Check sheet for the modelled part. Datum: model origin and axes. Units: mm. A direction names the side the tool comes from. Give positions to 0.01 mm unless a question says otherwise; leave off trailing zeros. Write each loop counter-clockwise with the first axis right and the second up, starting at its lowest first coordinate (ties: lowest second). Pieces come first, ordered by that corner, then holes. Notation, with made-up numbers: (1.25, 18) - (52.25, 18) arc R11 ccw to (52.25, 39) - close; hole circle Ø8 at (5, 56). An arc over 180 degrees is marked (long way). Return JSON: item names as keys, results as strings. Group by question number.
```python
from build123d import *

# Parameters (mm, degrees)
F0_R        = 19.5387268204
F1_DEPTH    = 101.6
F3_DEPTH    = 38.1
F5_DEPTH    = 25.4
F7_DEPTH    = 25.4
F8_T2_ANGLE = 300.1049055837
F8_T4_ANGLE = 131.5703123603


# Not quite as in the source:
# - a fillet or chamfer that OpenCascade refuses, or shapes differently, is made with other operations: its cross-section is extruded or revolved along the edge and cut away or added


with BuildPart() as f1:
    # F0 (on Right) → F1 (new body, symmetric)
    with BuildSketch(Plane.YZ):
        Circle(F0_R)
    extrude(amount=F1_DEPTH, both=True)

    # F2 (on Top) → F3 (cut)
    with BuildSketch(Plane.XY):
        Polygon((-49.3527501822, 13.7382084504), (-37.9295572639, 12.1708353981), (-49.3527501822, 22.1678428352), align=None)
    extrude(amount=-F3_DEPTH, mode=Mode.SUBTRACT)

    # F4 (on Top) → F5 (cut)
    with BuildSketch(Plane.XY):
        Polygon((-103.1729057431, 0), (-93.9432457089, -16.6200213134), (-87.8715068102, -10.7566714287), align=None)
        Polygon((22.2135502845, -11.3549903035), (22.2135502845, -20.1754160225), (26.9660595804, -20.1754160225), align=None)
        Polygon((-77.9622271657, 12.2874397784), (-86.7114588618, 22.1413038671), (-82.0683091879, 6.1605265364), (-65.0239139795, 12.2874397784), (-72.4504972355, 17.1812968249), align=None)
        Polygon((0, 22.1413038671), (-8.541457355, 12.2874397784), (0, 12.2874397784), align=None)
        Polygon((-27.3653976619, -12.4159986153), (-27.3653976619, -20.1754160225), (-12.2119756415, -16.6692733765), (-18.8832655549, -12.4159986153), align=None)
    extrude(amount=-F5_DEPTH, mode=Mode.SUBTRACT)

    # F6 (on Top) → F7 (cut)
    with BuildSketch(Plane.XY):
        Polygon((-32.052900187, -20.8235712349), (-20.0643315911, -22.1631750464), (-25.0567086041, -9.0359868482), (-35.0853319095, -12.8499542954), align=None)
        Polygon((23.2855007052, 4.9763009883), (30.9053044766, 17.5455939025), (23.2855007052, 13.3292628452), align=None)
        Polygon((-78.8187682629, 6.2337135896), (-83.6249142885, 11.739499867), (-95.4798087478, 0), (-87.3620659113, 0), align=None)
        Polygon((-32.4846748263, 17.5455939025), (-37.5734344125, 11.739499867), (-27.39591524, 11.739499867), align=None)
    extrude(amount=F7_DEPTH, mode=Mode.SUBTRACT)

    # F8: chamfer of 5.08 on 1 edges, made by hand

    # F8_s1 → F8_t2 (revolve, cut)
    with BuildSketch(Plane.XY):
        Polygon((-96.52, 19.5387268204), (-101.6, 14.4587268204), (-101.6, 19.5387268204), align=None)
    revolve(axis=Axis((-101.6, 0, 0), (1, 0, 0)), revolution_arc=F8_T2_ANGLE, mode=Mode.SUBTRACT)

    # F8_s3 → F8_t4 (revolve, cut)
    with BuildSketch(Plane(origin=(0, 0, 0), x_dir=(1, 0, 0), z_dir=(0, -0.7481420015, 0.6635386542))):
        Polygon((-96.52, -19.5387268204), (-101.6, -14.4587268204), (-101.6, -19.5387268204), align=None)
    revolve(axis=Axis((-101.6, 0, 0), (1, 0, 0)), revolution_arc=F8_T4_ANGLE, mode=Mode.SUBTRACT)


solid = f1.part
```
Item 1: Section check B-B on z = 4. Count the separate pieces of the cut face and the enclosed holes in it, plus the area to 3 significant figures.
Item 2: Depth check by flat-ended pin: pin 1 (7 mm diameter, centred on x = -6, z = -9, fed in from +Y); pin 2 (2 mm diameter, centred on x = -47, z = -7.5, fed in from -Y); pin 3 (2 mm diameter, centred on y = 11, z = 13, fed in from -X). Enter the tip coordinate at first touch or a pass-through.
Item 3: Section check A-A on x = -52. Record the cut outline in (y, z), plus the area to 3 significant figures.
Item 4: Access from +Z, -Z, +X, -X, +Y, -Y to the whole of each face (thin tool, end or side, straight path). Record for faces 1 (the face through (26, 11, 0)), 2 (the face through (-45, 16, 0)).
Item 5: Mould release check, pull along X, two halves, no side actions. Record for faces 3 (the face through (-101.6, 0, 0)), 4 (the face through (101.6, 0, 0)), 5 (the face through (-23.475, -13.194, 6.616)): +X half, -X half, draft (parallel to the pull), parting line (faces both ways), or undercut.
Item 6: Material ranges on line 1 along X through (y, z) = (9, 3.5); line 2 along X through (y, z) = (-16.5, 9.5); line 3 along Y through (x, z) = (-80, 10.5), recorded low to high. Write a range as from..to.
Reply:
{
 "1": {"separate pieces": "1", "enclosed holes": "3", "area": "7,500 mm²"},
 "2": {"pin 1": "y = 18.75", "pin 2": "y = -18.43", "pin 3": "x = -100.03"},
 "3": {"outline": "circle Ø39.08 at (0, 0)", "area": "1,200 mm²"},
 "4": {"face 1": "+Z", "face 2": "-Z"},
 "5": {"face 3": "-X half", "face 4": "+X half", "face 5": "undercut"},
 "6": {"line 1": "-101.6..-86.39, -81.23..23.29, 25.72..101.6", "line 2": "-97.02..-33.7, -22.22..101.6", "line 3": "-16.48..5.37, 7.59..16.48"}
}
